```python
from build123d import *

# Parameters (mm, degrees)
F3_R            = 7.5
F4_DEPTH        = 12.5
F4_COPIES_COUNT = 6
F6_D            = 2
F6_DEPTH        = 7
F6_TIP          = 0.600860619


# Not quite as in the source:
# - a fillet or chamfer that OpenCascade refuses, or shapes differently, is made with other operations: its cross-section is extruded or revolved along the edge and cut away or added
# - a pattern or mirror of a feature is missing from the dataset's text; its kind, count and spacing are read off the source's solid


with BuildPart() as f1:
    # F0 (on Front) → F1 (revolve)
    with BuildSketch(Plane.XZ):
        with BuildLine():
            Line((0, 8), (0, 5))
            Line((0, 5), (11.5, 4.4978991566))
            Line((11.5, 4.4978991566), (11.5, 28))
            ThreePointArc((11.5, 28), (12.0857864376, 29.4142135624), (13.5, 30))
            Line((13.5, 30), (14.5, 30))
            Line((14.5, 30), (14.5, 34))
            Line((14.5, 34), (-6.5, 34))
            Line((-6.5, 34), (-6.5, 30))
            Line((-6.5, 30), (1.5, 30))
            ThreePointArc((1.5, 30), (2.9142135624, 29.4142135624), (3.5, 28))
            Line((3.5, 28), (3.5, 10))
            ThreePointArc((3.5, 10), (2.9142135624, 8.5857864376), (1.5, 8))
            Line((1.5, 8), (0, 8))
        make_face()
    revolve(axis=Axis((5.75, 0, 0), (1, 0, 0)))

    # F2: chamfer of 0.25 on 7 edges, made by hand

    # F2_s1 → F2_t2 (revolve, cut)
    with BuildSketch(Plane.XZ):
        Polygon((-6.25, 34), (-6.5, 33.75), (-6.5, 34), align=None)
    revolve(axis=Axis((-6.5, 0, 0), (1, 0, 0)), mode=Mode.SUBTRACT)

    # F2_s3 → F2_t4 (revolve, cut)
    with BuildSketch(Plane.XZ):
        Polygon((-6.5, 30.25), (-6.25, 30), (-6.5, 30), align=None)
    revolve(axis=Axis((-6.5, 0, 0), (1, 0, 0)), mode=Mode.SUBTRACT)

    # F2_s5 → F2_t6 (revolve, cut)
    with BuildSketch(Plane.XZ):
        Polygon((14.25, 30), (14.5, 30.25), (14.5, 30), align=None)
    revolve(axis=Axis((14.5, 0, 0), (1, 0, 0)), mode=Mode.SUBTRACT)

    # F2_s7 → F2_t8 (revolve, cut)
    with BuildSketch(Plane.XZ):
        Polygon((14.5, 33.75), (14.25, 34), (14.5, 34), align=None)
    revolve(axis=Axis((14.5, 0, 0), (1, 0, 0)), mode=Mode.SUBTRACT)

    # F2_s9 → F2_t10 (revolve, cut)
    with BuildSketch(Plane.XZ):
        Polygon((0.25, 8), (0, 7.75), (0, 8), align=None)
    revolve(axis=Axis((0, 0, 0), (1, 0, 0)), mode=Mode.SUBTRACT)

    # F2_s11 → F2_t12 (revolve, cut)
    with BuildSketch(Plane.XZ):
        Polygon((0, 5.2393229356), (0.2390951532, 4.9895608802), (0, 5), align=None)
    revolve(axis=Axis((0, 0, 0), (1, 0, 0)), mode=Mode.SUBTRACT)

    # F2_s13 → F2_t14 (revolve, cut)
    with BuildSketch(Plane.XZ):
        Polygon((11.2390951532, 4.5092905082), (11.5, 4.7590525636), (11.5, 4.4978991566), align=None)
    revolve(axis=Axis((11.5, 0, 0), (1, 0, 0)), mode=Mode.SUBTRACT)

    # F3 (on Right) → F4 (cut, symmetric)
    with BuildSketch(Plane.YZ):
        with Locations((-19, 0)):
            Circle(F3_R)
    f4 = extrude(amount=F4_DEPTH, both=True, mode=Mode.SUBTRACT)

    # F4_copies: F4 ×6 about axis
    f4_copies_axis = Axis((0, 0, 0), (1, 0, 0))
    for i in range(1, F4_COPIES_COUNT):
        add(f4.rotate(f4_copies_axis, i * 360 / F4_COPIES_COUNT), mode=Mode.SUBTRACT)

    # F6
    with Locations(Plane.YZ.offset(14.5)):
        with Locations((0, -31.75), (0, -8.75)):
            Hole(F6_D / 2, depth=F6_DEPTH)
            with Locations((0, 0, -(F6_DEPTH + F6_TIP / 2))):  # 118° drill point
                Cone(0, F6_D / 2, F6_TIP, mode=Mode.SUBTRACT)


solid = f1.part
```
Can you work these out from the model? Positions are in its coordinate system, mm. A direction names the side the tool comes from. Give positions to 0.01 mm unless a question says otherwise; leave off trailing zeros. Answer in a Markdown table with one row per item.
1. Thinking about a two-plate mould opening in Z: for faces 1 (the flat face through (14.5, 17.3, 25.2)), 2 (the cylindrical face through (7.556, -26.493, 0.33)), 3 (the cylindrical face through (3.86, -28.67, 18.28)), which applies, released by +Z, released by -Z, zero draft, split by the parting line, or undercut?
Taken from the geometry:
| item | result |
|---|---|
| face 1 | zero draft |
| face 2 | undercut |
| face 3 | split by the parting line |
2. Which directions (+Z, -Z, +X, -X, +Y, -Y) give clear straight access to the entire face, cutting with the end or side of a thin tool? Please do faces 4 (the cylindrical face through (10.95, 0.13, -30.76)), 5 (the cylindrical face through (7.56, -13.53, 10.13)), 6 (the cylindrical face through (0.87, 7.81, -1.73)).
Taken from the geometry:
| item | result |
|---|---|
| face 4 | +X |
| face 5 | +X, -X |
| face 6 | -X |
3. If I drill on line 1 along Z through (x, y) = (0.25, 0); line 2 along Z through (x, y) = (9.5, 5); line 3 along Z through (x, y) = (13, 0), over which ranges is the centre line in solid material (lowest first)?
Taken from the geometry:
| item | result |
|---|---|
| line 1 | z = -34 to -30, -8 to -4.99, 4.99 to 8, 30 to 34 |
| line 2 | z = -33.63 to -22.45, -10.45 to 10.45, 22.45 to 33.63 |
| line 3 | z = -34 to -32.75, -30.75 to -29.94, 29.94 to 34 |
4. For pin 1 Ø1.2 at (y, z) = (0, -8.75) entering from +X; pin 2 Ø19.5 at (y, z) = (-9.5, -16.45) entering from +X; pin 3 Ø5 at (y, z) = (-17, 8.5) entering from -X; pin 4 Ø13.5 at (y, z) = (19, 0) entering from -X, each with a flat end and sliding along its axis, tell me the tip position at first contact or that it passes through.
Taken from the geometry:
| item | result |
|---|---|
| pin 1 | stops at x = 7.26 |
| pin 2 | stops at x = 11.64 |
| pin 3 | stops at x = 3.5 |
| pin 4 | passes through |
5. Suppose I cut it at A-A on x = 9. Count the separate pieces of the cut face and the enclosed holes in it, plus the area to 3 significant figures.
Taken from the geometry:
| item | result |
|---|---|
| separate pieces | 1 |
| enclosed holes | 9 |
| area | 2,500 mm² |
